Autodesk Inventor part; units mm, degrees
ref_plane "YZ Plane" through (0, 0, 0) normal (1, 0, 0) x (0, 1, 0)
ref_plane "XZ Plane" through (0, 0, 0) normal (0, 1, 0) x (-1, 0, 0)
ref_plane "XY Plane" through (0, 0, 0) normal (0, 0, 1) x (1, 0, 0)
sketch "Sketch1" plane through (0, 0, 0) normal (0, 1, 0) x (-1, 0, 0)
  point P0 (0, 0)
sketch "Sketch2" plane through (0, 0, 0) normal (0, 0, 1) x (1, 0, 0)
  circle A0 centre (0, -4.5) radius 0.9
  circle A1 centre (0, 4.5) radius 0.9
  circle A2 centre (0, 0) radius 2.0975
  line L0 (6.5, 7.5) -> (-6.5, 7.5)
  line L1 (-6.5, 7.5) -> (-6.5, -7.5)
  line L2 (-6.5, -7.5) -> (6.5, -7.5)
  line L3 (6.5, -7.5) -> (6.5, 7.5)
  dimension "d0" = 1.8
  dimension "d1" = 9
  dimension "d2" = 4.195
  dimension "d3" = 4.5
  dimension "d4" = 13
  dimension "d5" = 15
  dimension "d6" = 7.5
  dimension "d7" = 6.5
extrude "Extrusion1" add sketch "Sketch2" against normal blind 2
sketch "Sketch3" plane through (0, 0, -2) normal (0, 0, -1) x (-1, 0, 0)
  line L0 (6.5, 7.5) -> (-6.5, 7.5)
  line L1 (-6.5, 7.5) -> (-6.5, -7.5)
  line L2 (6.5, -7.5) -> (6.5, 7.5)
  line L3 (-6.5, -7.5) -> (6.5, -7.5)
  line L4 (-5.2, 6.2) -> (5.2, 6.2)
  line L5 (5.2, 6.2) -> (5.2, -6.2)
  line L6 (5.2, -6.2) -> (-5.2, -6.2)
  line L7 (-5.2, -6.2) -> (-5.2, 6.2)
  point P0 (0, 0)
  dimension "d10" = 1.3
  dimension "d11" = 1.3
  dimension "d12" = 1.3
  dimension "d13" = 1.3
extrude "Extrusion2" add sketch "Sketch3" along normal blind 7
sketch "Sketch4" plane through (-6.5, 7.5, 0) normal (0, 1, 0) x (1, 0, 0)
  line L0 (13, 9) -> (0, 9)
  line L1 (0, 9) -> (-10, 9)
  line L2 (-10, 9) -> (-10, 0)
  line L3 (0, 0) -> (13, 0)
  line L4 (-10, 0) -> (0, 0)
  line L5 (13, 0) -> (23, 0)
  line L6 (23, 0) -> (23, 9)
  line L7 (23, 9) -> (13, 9)
  line L8 (0, 0) -> (0, 9)
  line L9 (13, 0) -> (13, 9)
  circle A0 centre (-5.5, 4.5) radius 1.7
  circle A1 centre (18.5, 4.5) radius 1.7
  point P0 (6.5, 0)
  point P1 (-10, 4.5)
  point P2 (-5, 0)
  point P3 (18, 0)
  dimension "d16" = 3.4
  dimension "d17" = 10
  dimension "d22" = 4.5
  dimension "d23" = 4.5
extrude "Extrusion3" add sketch "Sketch4" against normal blind 3 contours L7 L6 L5 L9 | L8 L4 L2 L1
fillet "Fillet1" radius 2 2 edges at (-6.5, 4.5, -4.5) (6.5, 4.5, -4.5)
fillet "Fillet2" radius 4.5 4 edges at (-16.5, 6, 0) (-16.5, 6, -9) (16.5, 6, 0) (16.5, 6, -9)
sketch "Sketch5" plane through (-6.5, 4.5, 0) normal (0, -1, 0) x (1, 0, 0)
  circle A0 centre (18.5, -4.5) radius 1.7
  circle A1 centre (-5.5, -4.5) radius 1.7
  circle A2 centre (18.5, -4.5) radius 2.625
  circle A3 centre (-5.5, -4.5) radius 2.625
  point P0 (6.5, 0)
  dimension "d24" = 5.25
extrude "Extrusion4" cut sketch "Sketch5" against normal blind 1
fillet "Fillet3" radius 0.5 18 edges at (-6.5, -7.5, -4.5) (6.5, -7.5, -4.5) (-10.2502, 4.5, 0) (-15.1821, 4.5, -1.3179) (-16.5, 4.5, -4.5) (-10.2503, 4.5, -9) (-6.5, -2.5, -9) (-6.5, -2.5, 0) (10.2502, 4.5, 0) (15.1821, 4.5, -1.3179) (16.5, 4.5, -4.5) (10.2502, 4.5, -9) (6.5, -2.5, -9) (6.5, -2.5, 0) (0, -7.5, 0) (0, -7.5, -9) (0, 7.5, 0) (0, 7.5, -9)
fillet "Fillet4" radius 0.25 4 edges at (5.2, -6.2, -5.5) (-5.2, -6.2, -5.5) (5.2, 6.2, -5.5) (-5.2, 6.2, -5.5)
chamfer "Chamfer1" distance 0.25 angle 45 10 edges at (-2.0975, 0, -2) (-2.0975, 0, 0) (0, -6.2, -9) (5.1268, -6.1268, -9) (5.2, 0, -9) (5.1268, 6.1268, -9) (0, 6.2, -9) (-5.1268, 6.1268, -9) (-5.2, 0, -9) (-5.1268, -6.1268, -9)
sketch "Sketch6" plane through (0, 0, 0) normal (0, 0, 1) x (1, 0, 0)
  circle A0 centre (0, 4.5) radius 0.9
  circle A1 centre (0, 4.5) radius 1.575
  circle A2 centre (0, -4.5) radius 0.9
  circle A3 centre (0, -4.5) radius 1.575
  point P0 (0, 0)
  dimension "d32" = 3.15
extrude "Extrusion5" cut sketch "Sketch6" against normal blind 1
sketch "Sketch7" plane through (0, 4.5, -1) normal (0, 0, 1) x (1, 0, 0)
  circle A0 centre (0, 0) radius 0.9
  circle A1 centre (0, -9) radius 0.9
  point P0 (0, -4.5)
extrude "Extrusion6" [suppressed]
properties part number "v2motormount"
Model file for the job. Use its own axes, mm. A direction names the side the tool comes from. Round coordinates to 2 decimals unless told otherwise and drop trailing zeros. Loops run counter-clockwise (first coordinate to the right, second up) from the corner with the lowest first, then second, coordinate; pieces in that order, holes last. Notation, with made-up numbers: M 69,14.5 L 104,14.5 A10 cw 104,31.5 Z; hole C 22,8 d2. An arc over 180 degrees is marked long. Put each result on its own line as item: value. Start each with the question number.
Item 1: Cut at A-A (y = -4.5). List the corners of the cut face in (x, z) (3 decimals).
Item 2: Drop flat-ended pins along their axis: P1, Ø1, axis at y = 0.5, z = -3, coming from the -X side; P2, Ø3, axis at x = 12, z = -4.5, coming from the -Y side; P3, Ø2.5, axis at y = -1, z = -6, coming from the +X side; P4, Ø2.5, axis at x = -13, z = -5, coming from the -Y side. Give the stop position or say it passes through.
Item 3: Cut at D-D (y = 0). List the corners of the cut face in (x, z).
Item 4: 3-axis set-ups, long thin cutter, end or side, ignore diameter. For faces 1 (the face through (-9.8, 4.5, -6.3)), 2 (the face through (-5.2, 0, -5)), 3 (the face through (1, 4, -1)), 4 (the face through (-14.622, 4.993, -4.385)): which of +Z, -Z, +X, -X, +Y, -Y reach the whole face in a straight line?
Item 5: Cut at B-B (z = -3.75). Give the number of separate pieces and of enclosed holes in the cut face, then the cut area to 3 significant figures.
Item 6: Drill centre lines: line 1 along X through (y, z) = (6.65, -4.5); line 2 along Y through (x, z) = (0, -0.6) (1 decimal); line 3 along X through (y, z) = (-2, -5.5). Where is each one in solid material? Low to high.
Item 7: Mould opens along Z. For faces 5 (the face through (-10, 5.5, -4)), 6 (the face through (-2.4, -1.3, -2)), 7 (the face through (-6.5, -2, -4)) say: released by +Z, released by -Z, zero draft, split by the parting line, or undercut.
Answer block:
1. outline: M -6.5,-8.5 A0.5 ccw -6,-9 L -5.45,-9 L -5.2,-8.75 L -5.2,-2 L -0.9,-2 L -0.9,-1 L -1.575,-1 L -1.575,0 L -6,0 A0.5 ccw -6.5,-0.5 Z; M 0.9,-2 L 5.2,-2 L 5.2,-8.75 L 5.45,-9 L 6,-9 A0.5 ccw 6.5,-8.5 L 6.5,-0.5 A0.5 ccw 6,0 L 1.575,0 L 1.575,-1 L 0.9,-1 Z
2. P1: x = -6.5
2. P2: through
2. P3: x = 6.5
2. P4: y = 5.5
3. outline: M -6.5,-8.5 A0.5 ccw -6,-9 L -5.45,-9 L -5.2,-8.75 L -5.2,-2 L -2.35,-2 L -2.1,-1.75 L -2.1,-0.25 L -2.35,0 L -6,0 A0.5 ccw -6.5,-0.5 Z; M 2.1,-1.75 L 2.35,-2 L 5.2,-2 L 5.2,-8.75 L 5.45,-9 L 6,-9 A0.5 ccw 6.5,-8.5 L 6.5,-0.5 A0.5 ccw 6,0 L 2.35,0 L 2.1,-0.25 Z
4. face 1: +Z, -Z, -X, -Y
4. face 2: -Z
4. face 3: +Z
4. face 4: -Y
5. separate pieces: 3
5. enclosed holes: 1
5. area: 105 mm2
6. line 1: -16.5 to -13.7, -10.3 to 10.3, 13.7 to 16.5
6. line 2: -7.5 to -6.1, -2.9 to -2.1, 2.1 to 2.9, 6.1 to 7.5
6. line 3: -6.5 to -5.2, 5.2 to 6.5
7. face 5: undercut
7. face 6: released by -Z
7. face 7: zero draft
